```python
from build123d import *

# Parameters (mm, degrees)
BOSS_EXTRUDE1_DEPTH   = 82.55
BOSS_EXTRUDE2_REACH   = 38.963
SKETCH4_W             = 12.7
SKETCH4_H             = 82.55
F_6_CLEARANCE_HOLE1_D = 3.7973
SKETCH7_R             = 3.175
CUT_EXTRUDE1_DEPTH    = 31.613460512


with BuildPart() as part:
    # Sketch3 → Boss-Extrude1 (new body)
    with BuildSketch(Plane(origin=(0, 0, 0), x_dir=(1, 0, 0), z_dir=(0, 1, 0))):
        with BuildLine():
            Line((-43.815, -7.486539588), (-40.590360309, -7.486539588))
            ThreePointArc((-40.590360309, -7.486539588), (0, -41.275), (40.590360309, -7.486539588))
            Line((40.590360309, -7.486539588), (43.815, -7.486539588))
            ThreePointArc((43.815, -7.486539588), (0, -44.45), (-43.815, -7.486539588))
        make_face()
    extrude(amount=BOSS_EXTRUDE1_DEPTH)

    # Sketch4 → Boss-Extrude2 (add, up to next)
    with BuildSketch(Plane(origin=(0, 0, 7.486539588), x_dir=(-1, 0, 0), z_dir=(0, 0, -1)), mode=Mode.PRIVATE) as boss_extrude2_sk1:
        with Locations((-34.240360309, 41.275)):
            Rectangle(SKETCH4_W, SKETCH4_H)
    boss_extrude2_tool1 = extrude(boss_extrude2_sk1.sketch, amount=-BOSS_EXTRUDE2_REACH, mode=Mode.PRIVATE) - part.part
    add(boss_extrude2_tool1.solids().sort_by_distance((34.24036, 41.275, 7.48654))[0])
    # Sketch4 → Boss-Extrude2 (add, up to next)
    with BuildSketch(Plane(origin=(0, 0, 7.486539588), x_dir=(-1, 0, 0), z_dir=(0, 0, -1)), mode=Mode.PRIVATE) as boss_extrude2_sk2:
        with Locations((34.240360309, 41.275)):
            Rectangle(SKETCH4_W, SKETCH4_H)
    boss_extrude2_tool2 = extrude(boss_extrude2_sk2.sketch, amount=-BOSS_EXTRUDE2_REACH, mode=Mode.PRIVATE) - part.part
    add(boss_extrude2_tool2.solids().sort_by_distance((-34.24036, 41.275, 7.48654))[0])

    # #6 Clearance Hole1 (through all)
    with Locations(Plane(origin=(0, 0, 7.486539588), x_dir=(-1, 0, 0), z_dir=(0, 0, -1))):
        with Locations((-34.925, 77.47), (-34.925, 5.08), (34.925, 77.47), (34.925, 5.08)):
            Hole(F_6_CLEARANCE_HOLE1_D / 2)

    # Sketch7 → Cut-Extrude1 (cut, through all)
    with BuildSketch(Plane(origin=(0, 0, 13.836539588), x_dir=(-1, 0, 0), z_dir=(0, 0, -1))):
        with Locations((-34.925, 5.08)):
            Circle(SKETCH7_R)
        with Locations((34.925, 5.08)):
            Circle(SKETCH7_R)
        with Locations((34.925, 77.47)):
            Circle(SKETCH7_R)
        with Locations((-34.925, 77.47)):
            Circle(SKETCH7_R)
    extrude(amount=-CUT_EXTRUDE1_DEPTH, mode=Mode.SUBTRACT)


solid = part.part
```
Design review of the part built by this model. Coordinates are the model's own, in mm. A direction names the side the tool comes from. Coordinates: 2 decimals unless noted, no trailing zeros. Loops run counter-clockwise (first coordinate to the right, second up) from the corner with the lowest first, then second, coordinate; pieces in that order, holes last. Notation, with made-up numbers: (88, 21.5) -> (93, 21.5) arc R14 cw to (93, 30.5) -> close; hole circle Ø3 at (83.5, -3). An arc over 180 degrees is marked (long way). Answer as a JSON object with one key per item and string values.
Q1. Tool access review of faces 4 (the cylindrical face through (-36.43, 3.92, 10.71)), 5 (the cylindrical face through (-31.753, 77.61, 20.433)): name each direction out of +Z, -Z, +X, -X, +Y, -Y from which nothing blocks a thin tool from reaching the whole face with its end or side.
Answer block:
{"face 4": "+Z, -Z", "face 5": "+Z"}
Q2. Take a section at B-B on y = 5.08. Give the boundary of the cut face in (x, z) (3 decimals), plus the area to 3 significant figures.
Answer block:
{"outline": "(-43.815, 7.487) -> (-36.824, 7.487) -> (-36.824, 13.837) -> (-38.1, 13.837) -> (-38.1, 22.895) arc R44.45 ccw to start; (-33.026, 7.487) -> (-27.89, 7.487) -> (-27.89, 30.426) arc R41.275 cw to (27.89, 30.426) -> (27.89, 7.487) -> (33.026, 7.487) -> (33.026, 13.837) -> (31.75, 13.837) -> (31.75, 31.109) arc R44.45 ccw to (-31.75, 31.109) -> (-31.75, 13.837) -> (-33.026, 13.837) -> close; (36.824, 7.487) -> (43.815, 7.487) arc R44.45 ccw to (38.1, 22.895) -> (38.1, 13.837) -> (36.824, 13.837) -> close", "area": "527 mm^2"}
Q3. Take a section at C-C on z = 28.5. Give the boundary of the cut face in (x, y) (3 decimals).
Answer block:
{"outline": "(-34.111, 0) -> (-27.89, 0) -> (-27.89, 82.55) -> (-34.111, 82.55) -> (-34.111, 80.539) arc R3.175 cw to (-34.111, 74.401) -> (-34.111, 8.149) arc R3.175 cw to (-34.111, 2.011) -> close; (27.89, 0) -> (34.111, 0) -> (34.111, 2.011) arc R3.175 cw to (34.111, 8.149) -> (34.111, 74.401) arc R3.175 cw to (34.111, 80.539) -> (34.111, 82.55) -> (27.89, 82.55) -> close"}
Q4. Take a section at D-D on y = 41. Give the boundary of the cut face in (x, z) (3 decimals).
Answer block:
{"outline": "(-43.815, 7.487) -> (-27.89, 7.487) -> (-27.89, 30.426) arc R41.275 cw to (27.89, 30.426) -> (27.89, 7.487) -> (43.815, 7.487) arc R44.45 ccw to start"}
Q5. The part is to be moulded in two halves that separate along X. For faces 1 (the cylindrical face through (0.87, 40.7, 44.44)), 2 (the flat face through (27.89, 41, 19)), 3 (the flat face through (36, 42, 7.487)), say which applies: +X half, -X half, draft (parallel to the pull), parting line (faces both ways), or undercut.
Answer block:
{"face 1": "parting line", "face 2": "undercut", "face 3": "draft"}
Q6. To check wall thickness, follow L1, parallel to X at y = 77.47, z = 26.75; L2, parallel to Z at x = -37.5, y = 6; L3, parallel to X at y = 62.5, z = 28. State the ranges of each line that lie inside material, in increasing order.
Answer block:
{"L1": "x = -31.75 to -27.89, 27.89 to 31.75", "L2": "z = 7.49 to 13.84", "L3": "x = -34.52 to -27.89, 27.89 to 34.52"}
Q7. Clearance check with flat-ended pins moving along their axes: pin 1 Ø10 at (x, z) = (-31.5, 33.5) entering from +Y; pin 2 Ø4 at (y, z) = (23, 32.5) entering from +X (3 decimals); pin 3 Ø1.9 at (x, y) = (34, 76.5) entering from +Z; pin 4 Ø7.5 at (x, y) = (-34.925, 77.47) entering from +Z. State where each tip first meets the part, or that it passes through.
Answer block:
{"pin 1": "stops at y = 82.55", "pin 2": "stops at x = 32.335", "pin 3": "stops at z = 13.84", "pin 4": "stops at z = 31.68"}
Q8. Take a section at A-A on z = 16. Give the number of separate pieces and of enclosed holes in the cut face, plus the area to 3 significant figures.
Answer block:
{"separate pieces": "2", "enclosed holes": "4", "area": "2,120 mm^2"}
